```python
from build123d import *

# Parameters (mm, degrees)
AUFSATZ_LINEAR_AUSTRAGEN1_DEPTH = 1.4


with BuildPart() as part:
    # Skizze1 → Aufsatz-Linear austragen1 (new body)
    with BuildSketch(Plane(origin=(0, 0, 0), x_dir=(1, 0, 0), z_dir=(0, 1, 0))):
        Polygon((14.409630658, 25.21028647), (14.016111454, 25.259411872), (-14.016755293, 25.259390001), (-14.409855506, 25.210248977), (-14.705374814, 24.96453136), (-14.950840446, 24.669672719), (-15.000118678, 24.276547653), (-15.000218735, -28.257278341), (-14.95104056, -28.650375287), (-14.705137178, -28.945646353), (-14.410055621, -29.190951545), (-14.016949154, -29.240173804), (14.015942607, -29.240255039), (14.409480572, -29.191114015), (14.704562129, -28.945396398), (14.950465511, -28.650537758), (14.999712475, -28.257315834), (14.999781265, 24.276613266), (14.95060309, 24.669716461), (14.704274464, 24.964575102), align=None)
        with BuildLine():
            Line((11.462718603, -28.440255039), (-10.193671543, -28.440255039))
            ThreePointArc((-10.193671543, -28.440255039), (-10.547224933, -28.29380843), (-10.693671543, -27.940255039))
            Line((-10.693671543, -27.940255039), (-10.693671543, -27.530609999))
            ThreePointArc((-10.693671543, -27.530609999), (-10.840118152, -27.177056609), (-11.193671543, -27.030609999))
            Line((-11.193671543, -27.030609999), (-13.15, -27.030609999))
            Line((-13.15, -27.030609999), (-13.15, 23.169390001))
            Line((-13.15, 23.169390001), (13.15, 23.169390001))
            Line((13.15, 23.169390001), (13.15, -27.030609999))
            Line((13.15, -27.030609999), (12.462718603, -27.030609999))
            ThreePointArc((12.462718603, -27.030609999), (12.109165213, -27.177056609), (11.962718603, -27.530609999))
            Line((11.962718603, -27.530609999), (11.962718603, -27.940255039))
            ThreePointArc((11.962718603, -27.940255039), (11.816271994, -28.29380843), (11.462718603, -28.440255039))
        make_face(mode=Mode.SUBTRACT)
    extrude(amount=AUFSATZ_LINEAR_AUSTRAGEN1_DEPTH)


solid = part.part
```
Source: CAD feature listing. Evaluate the final solid. Frame: model axes, mm. A direction names the side the tool comes from. Give positions to 0.01 mm unless a question says otherwise; leave off trailing zeros. Order: outer loops, then holes, each group sorted by start corner. A loop starts at its lowest first (then second) coordinate and runs counter-clockwise, first axis right, second up.
(1) Section query C-C (z = 3). Return the cut outline in (x, y).
(2) Pull-direction query (X, two-part tool) for faces 1 (the face through (-13.4, 0, -4.2)), 2 (the face through (-13.15, 1, 2)); classes: +X half, -X half, draft (parallel to the pull), parting line (faces both ways), or undercut.
(3) Section query B-B (x = -8.5). Return the cut outline in (y, z), plus the area to 3 significant figures.
(4) Access query for faces 3 (the face through (-12, 1, 27.031)), 4 (the face through (0, 1, -25.259)). Directions: +Z, -Z, +X, -X, +Y, -Y. A direction counts if a zero-diameter tool reaches every point of the face in a straight line with its end or side. Return the directions, or none.
(5) Material intervals for line 1 along X through (y, z) = (0.9, -20); line 2 along Z through (x, y) = (-0.5, 0.55); line 3 along Z through (x, y) = (-12.5, 0.65), sorted ascending.
Outcome:
1. outline: (-15, 0) - (-13.15, 0) - (-13.15, 1.4) - (-15, 1.4) - close; (13.15, 0) - (15, 0) - (15, 1.4) - (13.15, 1.4) - close
2. face 1: draft
2. face 2: undercut
3. outline: (0, -25.26) - (1.4, -25.26) - (1.4, -23.17) - (0, -23.17) - close; (0, 28.44) - (1.4, 28.44) - (1.4, 29.24) - (0, 29.24) - close
3. area: 4.05 mm2
4. face 3: +Y, -Y
4. face 4: -Z, +X, -X, +Y, -Y
5. line 1: x = -15 to -13.15, 13.15 to 15
5. line 2: z = -25.26 to -23.17, 28.44 to 29.24
5. line 3: z = -25.26 to -23.17, 27.03 to 29.24
